from build123d import *

# Parameters (mm, degrees)
SKETCH1_W                    = 29
SKETCH1_H                    = 47
BASE_FLANGE1_DEPTH           = 1.5
EDGE_FLANGE1_STRIP_W         = 10
EDGE_FLANGE1_STRIP_H         = 1.5
EDGE_FLANGE1_STRIP_CUT_DEPTH = 47
EDGE_FLANGE1_DEPTH           = 47
EDGE_FLANGE2_STRIP_W         = 10
EDGE_FLANGE2_STRIP_H         = 1.5
EDGE_FLANGE2_STRIP_CUT_DEPTH = 47
EDGE_FLANGE2_DEPTH           = 47
SKETCH12_R                   = 1.6
CUT_EXTRUDE1_DEPTH           = 10
SKETCH13_R                   = 1.325
CUT_EXTRUDE2_DEPTH           = 62.012293843
FILLET1_R                    = 5


# Sheet-metal steps are written as plain solids
with BuildPart() as part:
    # Sketch1 → Base-Flange1 (new body)
    with BuildSketch(Plane(origin=(0, 0, 0), x_dir=(1, 0, 0), z_dir=(0, 1, 0))):
        Rectangle(SKETCH1_W, SKETCH1_H)
    extrude(amount=BASE_FLANGE1_DEPTH)

    # Edge-Flange1 strip (across the edge) → Edge-Flange1 strip cut (cut)
    with BuildSketch(Plane(origin=(14.5, 1.5, 23.5), x_dir=(-1, 0, 0), z_dir=(0, 0, -1))):
        with Locations((-3, -0.75)):
            Rectangle(EDGE_FLANGE1_STRIP_W, EDGE_FLANGE1_STRIP_H)
    edge_flange1_strip_cut = extrude(amount=EDGE_FLANGE1_STRIP_CUT_DEPTH, mode=Mode.SUBTRACT)

    # Edge-Flange1 section (across the edge) → Edge-Flange1 (add)
    with BuildSketch(Plane(origin=(14.5, 1.5, 23.5), x_dir=(-1, 0, 0), z_dir=(0, 0, -1))):
        with BuildLine():
            Line((-1.5, 2), (-1.5, 36))
            Line((-1.5, 36), (0, 36))
            Line((0, 36), (0, 2))
            ThreePointArc((0, 2), (0.585786438, 0.585786438), (2, 0))
            Line((2, 0), (2, -1.5))
            ThreePointArc((2, -1.5), (-0.474873734, -0.474873734), (-1.5, 2))
        make_face()
    edge_flange1 = extrude(amount=EDGE_FLANGE1_DEPTH)

    # Mirror1: Edge-Flange1 strip cut, Edge-Flange1 across plane
    add(edge_flange1_strip_cut.mirror(Plane(origin=(0, 0, 0), x_dir=(0, 0, 1), z_dir=(1, 0, 0))), mode=Mode.SUBTRACT)
    add(edge_flange1.mirror(Plane(origin=(0, 0, 0), x_dir=(0, 0, 1), z_dir=(1, 0, 0))))

    # Edge-Flange2 strip (across the edge) → Edge-Flange2 strip cut (cut)
    with BuildSketch(Plane(origin=(-16, 37.5, 23.5), x_dir=(0, -1, 0), z_dir=(0, 0, -1))):
        with Locations((-1.5, -0.75)):
            Rectangle(EDGE_FLANGE2_STRIP_W, EDGE_FLANGE2_STRIP_H)
    edge_flange2_strip_cut = extrude(amount=EDGE_FLANGE2_STRIP_CUT_DEPTH, mode=Mode.SUBTRACT)

    # Edge-Flange2 section (across the edge) → Edge-Flange2 (add)
    with BuildSketch(Plane(origin=(-16, 37.5, 23.5), x_dir=(0, -1, 0), z_dir=(0, 0, -1))):
        with BuildLine():
            Line((0, 2), (0, 10))
            Line((0, 10), (1.5, 10))
            Line((1.5, 10), (1.5, 2))
            ThreePointArc((1.5, 2), (2.085786438, 0.585786438), (3.5, 0))
            Line((3.5, 0), (3.5, -1.5))
            ThreePointArc((3.5, -1.5), (1.025126266, -0.474873734), (0, 2))
        make_face()
    edge_flange2 = extrude(amount=EDGE_FLANGE2_DEPTH)

    # Mirror2: Edge-Flange2 strip cut, Edge-Flange2 across plane
    add(edge_flange2_strip_cut.mirror(Plane(origin=(0, 0, 0), x_dir=(0, 0, 1), z_dir=(1, 0, 0))), mode=Mode.SUBTRACT)
    add(edge_flange2.mirror(Plane(origin=(0, 0, 0), x_dir=(0, 0, 1), z_dir=(1, 0, 0))))

    # Sketch12 → Cut-Extrude1 (cut)
    with BuildSketch(Plane(origin=(0, 37.5, 0), x_dir=(1, 0, 0), z_dir=(0, 1, 0))):
        with Locations(Location((21.5, 15, 0), (0, 0, 270))):
            Circle(SKETCH12_R)
        with Locations(Location((-21.5, 15, 0), (0, 0, 270))):
            Circle(SKETCH12_R)
        with Locations(Location((-21.5, -15, 0), (0, 0, 270))):
            Circle(SKETCH12_R)
        with Locations(Location((21.5, -15, 0), (0, 0, 270))):
            Circle(SKETCH12_R)
    extrude(amount=-CUT_EXTRUDE1_DEPTH, mode=Mode.SUBTRACT)

    # Sketch13 → Cut-Extrude2 (cut, through all)
    with BuildSketch(Plane(origin=(16, 0, 0), x_dir=(0, 0, -1), z_dir=(1, 0, 0))):
        with Locations(Location((-4, 26, 0), (0, 0, 270))):
            Circle(SKETCH13_R)
        with Locations(Location((-4, 14, 0), (0, 0, 270))):
            Circle(SKETCH13_R)
    extrude(amount=-CUT_EXTRUDE2_DEPTH, mode=Mode.SUBTRACT)

    # Fillet1
    fillet1_edges = [part.edges().sort_by_distance(p)[0] for p in [
        (-26, 36.75, 23.5),
        (-26, 36.75, -23.5),
        (26, 36.75, -23.5),
        (26, 36.75, 23.5),
    ]]
    fillet(fillet1_edges, radius=FILLET1_R)


solid = part.part
Geometry check sheet. Reference: the model listing, model coordinates, mm. A direction names the side the tool comes from. Coordinates: 2 decimals unless noted, no trailing zeros. Order: outer loops, then holes, each group sorted by start corner. A loop starts at its lowest first (then second) coordinate and runs counter-clockwise, first axis right, second up. Notation, with made-up numbers: (-26, -1.75) - (0, -1.75) arc R19 ccw to (0, 8.25) - close; hole circle Ø9 at (69.5, 83.5). An arc over 180 degrees is marked (long way). Answer in a Markdown table with one row per item. Add a question column.
1) Release check for a two-part mould opening along Y. For faces 4 (the flat face through (22, 37.5, 0)), 5 (the cylindrical face through (15.26, 24.776, 4.507)), 6 (the cylindrical face through (22.58, 36.76, -16.18)), 7 (the flat face through (-22, 36, 0)) record: +Y half, -Y half, draft (parallel to the pull), parting line (faces both ways), or undercut.
2) Cross-section at A-A, the plane z = -15. Record the cut outline in (x, y).
3) Cross-section at C-C, the plane z = 12. Record the cut outline in (x, y), then the cut area to 3 significant figures.
4) Set-up check for faces 1 (the cylindrical face through (-24.5, 36.74, 22.07)), 2 (the flat face through (16, 19, 0)), 3 (the cylindrical face through (-15.5, 36.45, 0.33)): record each of +Z, -Z, +X, -X, +Y, -Y from which the full face is reachable in a straight line by a thin tool's end or side.
5) Cross-section at D-D, the plane z = 4. State how many separate pieces and enclosed holes the cut face has, then the cut area to 3 significant figures.
6) Gauge pin test, flat ends, axial feed: P1, Ø2, axis at y = 14, z = 4, coming from the +X side; P2, Ø3, axis at y = 8, z = -13, coming from the -X side; P3, Ø7.5, axis at x = -4, z = -4, coming from the +Y side; P4, Ø9, axis at x = 23.5, z = -5.5, coming from the -Y side. Record the tip position at first contact, or that the pin passes through.
7) Material ranges on line 1 along Z through (x, y) = (15.1, 26) (3 decimals); line 2 along X through (y, z) = (3.5, 3.5); line 3 along Y through (x, z) = (-15.4, 4) (3 decimals), recorded low to high. Write a range as [from, to].
8) Cross-section at B-B, the plane y = 23.5. Record the cut outline in (x, z).
Check result:
| question | item | result |
|---|---|---|
| 1 | face 4 | +Y half |
| 1 | face 5 | undercut |
| 1 | face 6 | draft |
| 1 | face 7 | -Y half |
| 2 | outline | (-26, 36) - (-23.1, 36) - (-23.1, 37.5) - (-26, 37.5) - close; (-19.9, 36) - (-18, 36) arc R2 cw to (-16, 34) - (-16, 3.5) arc R3.5 ccw to (-12.5, 0) - (12.5, 0) arc R3.5 ccw to (16, 3.5) - (16, 34) arc R2 cw to (18, 36) - (19.9, 36) - (19.9, 37.5) - (18, 37.5) arc R3.5 ccw to (14.5, 34) - (14.5, 3.5) arc R2 cw to (12.5, 1.5) - (-12.5, 1.5) arc R2 cw to (-14.5, 3.5) - (-14.5, 34) arc R3.5 ccw to (-18, 37.5) - (-19.9, 37.5) - close; (23.1, 36) - (26, 36) - (26, 37.5) - (23.1, 37.5) - close |
| 3 | outline | (-26, 36) - (-18, 36) arc R2 cw to (-16, 34) - (-16, 3.5) arc R3.5 ccw to (-12.5, 0) - (12.5, 0) arc R3.5 ccw to (16, 3.5) - (16, 34) arc R2 cw to (18, 36) - (26, 36) - (26, 37.5) - (18, 37.5) arc R3.5 ccw to (14.5, 34) - (14.5, 3.5) arc R2 cw to (12.5, 1.5) - (-12.5, 1.5) arc R2 cw to (-14.5, 3.5) - (-14.5, 34) arc R3.5 ccw to (-18, 37.5) - (-26, 37.5) - close |
| 3 | area | 179 mm² |
| 4 | face 1 | +Z, -X, +Y, -Y |
| 4 | face 2 | +Z, -Z, +X, -Y |
| 4 | face 3 | +Z, -Z, +Y |
| 5 | separate pieces | 5 |
| 5 | enclosed holes | 0 |
| 5 | area | 163 mm² |
| 6 | P1 | passes through |
| 6 | P2 | stops at x = -16 |
| 6 | P3 | stops at y = 1.5 |
| 6 | P4 | stops at y = 36 |
| 7 | line 1 | z = [-23.5, 2.675], [5.325, 23.5] |
| 7 | line 2 | x = [-16, -14.5], [14.5, 16] |
| 7 | line 3 | y = [1.54, 12.675], [15.325, 24.675], [27.325, 36.343] |
| 8 | outline | (-16, -23.5) - (-14.5, -23.5) - (-14.5, 23.5) - (-16, 23.5) - close; (14.5, -23.5) - (16, -23.5) - (16, 23.5) - (14.5, 23.5) - close |
